Input: part model. Units: mm. Frame: model coordinates. Face numbers are marked on the shaded views. A direction names the side the tool comes from. Give positions to 0.01 mm unless a question says otherwise; leave off trailing zeros. Loops run counter-clockwise (first coordinate to the right, second up) from the corner with the lowest first, then second, coordinate; pieces in that order, holes last.
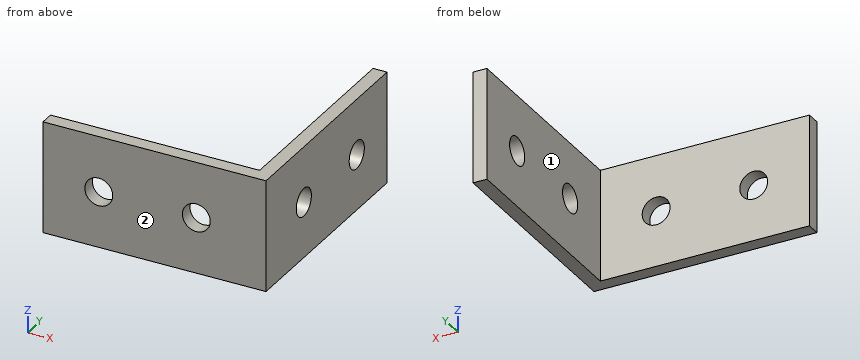
Autodesk Inventor part; units mm, degrees
ref_plane "YZ Plane" through (0, 0, 0) normal (1, 0, 0) x (0, 1, 0)
ref_plane "XZ Plane" through (0, 0, 0) normal (0, 1, 0) x (-1, 0, 0)
ref_plane "XY Plane" through (0, 0, 0) normal (0, 0, 1) x (1, 0, 0)
sketch "Sketch1" plane through (0, 0, 0) normal (0, 0, 1) x (1, 0, 0)
  line L0 (0, 0) -> (-50.8, 0)
  line L1 (-50.8, 0) -> (-50.8, 3.175)
  line L2 (-50.8, 3.175) -> (-3.175, 3.175)
  line L3 (-3.175, 3.175) -> (-3.175, 50.8)
  line L4 (-3.175, 50.8) -> (0, 50.8)
  line L5 (0, 50.8) -> (0, 0)
  dimension "d0" = 3.175
  dimension "d1" = 50.8
extrude "Extrusion1" add sketch "Sketch1" along normal blind 25.4
sketch "Sketch2" plane through (-50.8, 0, 0) normal (0, -1, 0) x (1, 0, 0)
  line L0 (50.8, 0) -> (50.8, 25.4)
  line L1 (0, 25.4) -> (50.8, 25.4)
  point P0 (12.7, 12.7)
  point P1 (34.925, 12.7)
  dimension "d4" = 15.875
  dimension "d5" = 22.225
  dimension "d6" = 12.7
  dimension "d7" = 12.7
hole "Hole1" at (-38.1, 0, 12.7) at (-15.875, 0, 12.7) direction (0, 1, 0) diameter 6.35 end through all
sketch "Sketch3" plane through (0, 0, 0) normal (1, 0, 0) x (0, 0, -1)
  line L0 (0, 50.8) -> (0, 0)
  line L1 (-15.875, 3.175) -> (-9.525, 3.175)
  point P0 (-12.7, 15.875)
  point P1 (-12.7, 38.1)
  dimension "d15" = 12.7
  dimension "d16" = 12.7
  dimension "d17" = 12.7
  dimension "d18" = 22.225
hole "Hole2" at (0, 15.875, 12.7) at (0, 38.1, 12.7) direction (-1, 0, 0) diameter 6.35 end through all
properties part number "2x1 angle bracket" material "Aluminum 6061"
(1) Cut plane B-B (x = -38.1). Return the cut outline in (y, z) (3 decimals).
Values follow:
outline: (0, 0) - (3.175, 0) - (3.175, 9.525) - (0, 9.525) - close; (0, 15.875) - (3.175, 15.875) - (3.175, 25.4) - (0, 25.4) - close
(2) Reachability of the marked faces 1 and 2 from +Z, -Z, +X, -X, +Y, -Y: full face, straight path, thin tool, end or side. Return the list, or none.
Values follow:
face 1: +Z, -Z, -X, +Y
face 2: +Z, -Z, +X, -X, -Y
(3) Cut plane D-D (z = 3). Return the cut outline in (x, y) (3 decimals), and give its area (4 significant figures).
Values follow:
outline: (-50.8, 0) - (0, 0) - (0, 50.8) - (-3.175, 50.8) - (-3.175, 3.175) - (-50.8, 3.175) - close
area: 312.5 mm2
(4) Cut plane A-A (z = 12.7). Return the cut outline in (x, y) (3 decimals).
Values follow:
outline: (-50.8, 0) - (-41.275, 0) - (-41.275, 3.175) - (-50.8, 3.175) - close; (-34.925, 0) - (-19.05, 0) - (-19.05, 3.175) - (-34.925, 3.175) - close; (-12.7, 0) - (0, 0) - (0, 12.7) - (-3.175, 12.7) - (-3.175, 3.175) - (-12.7, 3.175) - close; (-3.175, 19.05) - (0, 19.05) - (0, 34.925) - (-3.175, 34.925) - close; (-3.175, 41.275) - (0, 41.275) - (0, 50.8) - (-3.175, 50.8) - close
(5) Pin query (flat end, axial travel): pin 1 Ø1 at (x, z) = (-45.5, 11.5) entering from -Y; pin 2 Ø2 at (x, z) = (-16, 14.5) entering from +Y; pin 3 Ø7.5 at (y, z) = (18.5, 14) entering from -X (3 decimals); pin 4 Ø6 at (x, z) = (-14.5, 17.5) entering from +Y (3 decimals). Return the tip coordinate at first contact, or that it passes through.
Values follow:
pin 1: stops at y = 0
pin 2: passes through
pin 3: stops at x = -3.175
pin 4: stops at y = 3.175
(6) Ray query, probe 1 along Y at (x, z) = (-2.1, 12.7) (3 decimals); probe 2 along X at (y, z) = (2.4, 12.7) (3 decimals); probe 3 along Z at (x, y) = (-38.1, 1.5) (3 decimals). Return the intervals inside material, ascending.
Values follow:
probe 1: y = 0 to 12.7, 19.05 to 34.925, 41.275 to 50.8
probe 2: x = -50.8 to -41.275, -34.925 to -19.05, -12.7 to 0
probe 3: z = 0 to 9.525, 15.875 to 25.4
(7) Cut plane C-C (y = 38.1). Return the cut outline in (x, z) (3 decimals), and give its area (3 significant figures).
Values follow:
outline: (-3.175, 0) - (0, 0) - (0, 9.525) - (-3.175, 9.525) - close; (-3.175, 15.875) - (0, 15.875) - (0, 25.4) - (-3.175, 25.4) - close
area: 60.5 mm2
